Check sheet for the modelled part. Datum: model origin and axes. Units: mm. A direction names the side the tool comes from. Coordinates: 2 decimals unless noted, no trailing zeros. Order: outer loops, then holes, each group sorted by start corner. A loop starts at its lowest first (then second) coordinate and runs counter-clockwise, first axis right, second up.
1. Cross-section at D-D (x = 37). Enter the section's corners in (y, z), then the cut area to 3 significant figures.
2. Draft check along Y on faces 1 (the flat face through (42, 36, -1)), 2 (the flat face through (30, 23, -3)), 3 (the flat face through (40, 46, -1)), 4 (the flat face through (30, 37, -1)). Enter one of: released by +Y, released by -Y, zero draft, split by the parting line, or undercut.
3. Gauge pin test, flat ends, axial feed: pin 1 Ø1.5 at (x, z) = (50, -1.5) entering from -Y; pin 2 Ø0.9 at (x, z) = (13.5, -2) entering from +Y; pin 3 Ø0.9 at (y, z) = (1, -2) entering from -X. Record the tip position at first contact, or that the pin passes through.
4. Cross-section at B-B (y = 10.65). Enter the section's corners in (x, z).
5. Cross-section at A-A (x = 5). Enter the section's corners in (y, z).
6. Thickness scan on line 1 (X direction, y = 36.5, z = -2); line 2 (Y direction, x = 38, z = -1.6); line 3 (X direction, y = 9.5, z = -1.3). Record the ranges inside material, lowest first.
7. Cross-section at C-C (z = -0.55). Enter the section's corners in (x, y).
8. Set-up check for faces 5 (the flat face through (18, 2, -1)), 6 (the flat face through (42, 1, -1)), 7 (the flat face through (30, 34, -1)), 8 (the flat face through (52, 43, -1)): record each of +Z, -Z, +X, -X, +Y, -Y from which the full face is reachable in a straight line by a thin tool's end or side.
Autodesk Inventor part; units mm, degrees
ref_plane "YZ Plane" through (0, 0, 0) normal (1, 0, 0) x (0, 1, 0)
ref_plane "XZ Plane" through (0, 0, 0) normal (0, 1, 0) x (-1, 0, 0)
ref_plane "XY Plane" through (0, 0, 0) normal (0, 0, 1) x (1, 0, 0)
sketch "Sketch1" plane through (0, 0, 0) normal (0, 0, 1) x (1, 0, 0)
  line L0 (42, 0) -> (60, 0)
  line L1 (42, 0) -> (18, 0)
  line L2 (0, 0) -> (18, 0)
  line L3 (60, 0) -> (60, 3) construction
  line L4 (0, 0) -> (0, 3) construction
  line L5 (24, 16) -> (47, 16) construction
  line L6 (60, 0) -> (0, 0)
  line L7 (0, 0) -> (0, 40)
  line L8 (0, 40) -> (60, 40)
  line L9 (60, 40) -> (60, 0)
  line L10 (52, 40) -> (28, 40)
  line L11 (28, 40) -> (28, 46)
  line L12 (28, 46) -> (52, 46)
  line L13 (52, 46) -> (52, 40)
  line L14 (42, 3) -> (42, 0) construction
  line L15 (18, 0) -> (18, 3) construction
  line L16 (42, 34) -> (18, 34)
  line L17 (18, 34) -> (18, 37)
  line L18 (18, 37) -> (42, 37)
  line L19 (42, 37) -> (42, 34)
  dimension "d0" = 40
  dimension "d1" = 8
  dimension "d2" = 24
  dimension "d3" = 6
  dimension "d4" = 3
  dimension "d5" = 3
  dimension "d6" = 24
extrude "Extrusion1" add sketch "Sketch1" against normal blind 3
sketch "Sketch2" plane through (0, 0, 0) normal (0, 0, 1) x (1, 0, 0)
  line L0 (42, 0) -> (42, 3)
  line L1 (60, 3) -> (42, 3)
  line L2 (60, 0) -> (60, 3)
  line L3 (60, 0) -> (42, 0)
  line L4 (18, 3) -> (18, 0)
  line L5 (18, 0) -> (0, 0)
  line L6 (0, 0) -> (0, 3)
  line L7 (18, 3) -> (0, 3)
extrude "Extrusion2" cut sketch "Sketch2" against normal blind 3
sketch "Sketch3" plane through (0, 0, -3) normal (0, 0, -1) x (-1, 0, 0)
  arc A0 (-3.15, 12.05) -> (-6.85, 12.05) centre (-5, 12.05) ccw construction
  line L0 (-3.15, 12.05) -> (-3.15, 9.25) construction
  arc A1 (-6.85, 9.25) -> (-3.15, 9.25) centre (-5, 9.25) ccw construction
  line L1 (-6.85, 9.25) -> (-6.85, 12.05) construction
  arc A2 (-9, 17.6) -> (-10, 16.6) centre (-9, 16.6) ccw construction
  line L2 (-10, 16.6) -> (-10, 4) construction
  line L3 (-10, 4) -> (0, 4) construction
  line L4 (0, 4) -> (0, 16.6) construction
  arc A3 (0, 16.6) -> (-1, 17.6) centre (-1, 16.6) ccw construction
  line L5 (-1, 17.6) -> (-9, 17.6) construction
  arc A4 (-53.15, 12.05) -> (-56.85, 12.05) centre (-55, 12.05) ccw construction
  line L6 (-53.15, 12.05) -> (-53.15, 9.25) construction
  arc A5 (-56.85, 9.25) -> (-53.15, 9.25) centre (-55, 9.25) ccw construction
  line L7 (-56.85, 9.25) -> (-56.85, 12.05) construction
  arc A6 (-59, 17.6) -> (-60, 16.6) centre (-59, 16.6) ccw construction
  line L8 (-60, 16.6) -> (-60, 4) construction
  line L9 (-60, 4) -> (-50, 4) construction
  line L10 (-50, 4) -> (-50, 16.6) construction
  arc A7 (-50, 16.6) -> (-51, 17.6) centre (-51, 16.6) ccw construction
  line L11 (-51, 17.6) -> (-59, 17.6) construction
  line L12 (-5, 9.25) -> (-5, 12.05) construction
  line L13 (-55, 9.25) -> (-55, 12.05) construction
  circle A8 centre (-5, 10.65) radius 1.85
  circle A9 centre (-55, 10.65) radius 1.85
  point P0 (0, 0)
extrude "Extrusion3" cut sketch "Sketch3" against normal blind 22.4
properties part number "Pan base top side bars"
Data:
1. outline: (0, -3) - (34, -3) - (34, 0) - (0, 0) - close; (37, -3) - (46, -3) - (46, 0) - (37, 0) - close
1. area: 129 mm2
2. face 1: undercut
2. face 2: zero draft
2. face 3: released by +Y
2. face 4: undercut
3. pin 1: stops at y = 3
3. pin 2: stops at y = 40
3. pin 3: stops at x = 18
4. outline: (0, -3) - (3.15, -3) - (3.15, 0) - (0, 0) - close; (6.85, -3) - (53.15, -3) - (53.15, 0) - (6.85, 0) - close; (56.85, -3) - (60, -3) - (60, 0) - (56.85, 0) - close
5. outline: (3, -3) - (8.8, -3) - (8.8, 0) - (3, 0) - close; (12.5, -3) - (40, -3) - (40, 0) - (12.5, 0) - close
6. line 1: x = 0 to 18, 42 to 60
6. line 2: y = 0 to 34, 37 to 46
6. line 3: x = 0 to 3.55, 6.45 to 53.55, 56.45 to 60
7. outline: (0, 3) - (18, 3) - (18, 0) - (42, 0) - (42, 3) - (60, 3) - (60, 40) - (52, 40) - (52, 46) - (28, 46) - (28, 40) - (0, 40) - close; hole circle Ø3.7 at (5, 10.65); hole (18, 34) - (42, 34) - (42, 37) - (18, 37) - close; hole circle Ø3.7 at (55, 10.65)
8. face 5: +Z, -Z, -X, -Y
8. face 6: +Z, -Z, +X, -Y
8. face 7: +Z, -Z
8. face 8: +Z, -Z, +X, +Y
